from build123d import *

# Parameters (mm, degrees)
F0_W      = 25
F0_H      = 25
F1_DEPTH  = 25
F3_DEPTH  = 25
F9_W      = 25
F9_H      = 25
F10_DEPTH = 25
F11_R     = 5
F12_R     = 5


with BuildPart() as f1:
    # F0 (on Top) → F1 (new body)
    with BuildSketch(Plane.XY):
        Polygon((38.8634320385, -116.9341091547), (38.8634320385, -141.9341091547), (288.8634320385, -141.9341091547), (288.8634320385, 183.0658908453), (38.8634320385, 183.0658908453), (38.8634320385, 158.0658908453), (38.8634320385, 133.0658908453), (38.8634320385, 108.0658908453), (38.8634320385, 83.0658908453), (38.8634320385, 58.0658908453), (38.8634320385, 33.0658908453), (38.8634320385, 8.0658908453), (38.8634320385, -16.9341091547), (38.8634320385, -41.9341091547), (38.8634320385, -66.9341091547), (38.8634320385, -91.9341091547), align=None)
        with Locations((26.3634320385, -129.4341091547)):
            Rectangle(F0_W, F0_H)
        with Locations((26.3634320385, -79.4341091547)):
            Rectangle(F0_W, F0_H)
        with Locations((26.3634320385, -29.4341091547)):
            Rectangle(F0_W, F0_H)
        with Locations((26.3634320385, 20.5658908453)):
            Rectangle(F0_W, F0_H)
        with Locations((26.3634320385, 70.5658908453)):
            Rectangle(F0_W, F0_H)
        with Locations((26.3634320385, 120.5658908453)):
            Rectangle(F0_W, F0_H)
        with Locations((26.3634320385, 170.5658908453)):
            Rectangle(F0_W, F0_H)
    extrude(amount=F1_DEPTH)

    # F2 (on face) → F3 (cut)
    with BuildSketch(Plane.XZ.offset(141.9341091547)):
        Polygon((208.8634320385, 25), (203.8634320385, 0), (228.8634320385, 0), (223.8634320385, 25), align=None)
    extrude(amount=-F3_DEPTH, mode=Mode.SUBTRACT)

    # F8: F1 across plane


with BuildPart() as f1_1:
    add(f1.part)
    add(f1.part.mirror(Plane(origin=(288.8634320385, 20.5658908453, 0), x_dir=(0, 0, 1), z_dir=(0, 1, 0))), mode=Mode.INTERSECT)

    # F9 (on face) → F10 (cut)
    with BuildSketch(Plane(origin=(0, 0, 0), x_dir=(1, 0, 0), z_dir=(0, 0, -1))):
        with Locations((183.8634320385, -145.5658908453)):
            Rectangle(F9_W, F9_H)
        with Locations((183.8634320385, -95.5658908453)):
            Rectangle(F9_W, F9_H)
        with Locations((183.8634320385, -45.5658908453)):
            Rectangle(F9_W, F9_H)
        with Locations((183.8634320385, 4.4341091547)):
            Rectangle(F9_W, F9_H)
        with Locations((183.8634320385, 54.4341091547)):
            Rectangle(F9_W, F9_H)
        with Locations((183.8634320385, 104.4341091547)):
            Rectangle(F9_W, F9_H)
    extrude(amount=-F10_DEPTH, mode=Mode.SUBTRACT)

    # F11
    f11_edges = [f1_1.edges().sort_by_distance(p)[0] for p in [
        (108.863432, -141.934109, 0),
        (111.363432, -141.934109, 25),
        (256.363432, -141.934109, 25),
        (258.863432, -141.934109, 0),
    ]]
    fillet(f11_edges, radius=F11_R)

    # F12
    f12_edges = [f1_1.edges().sort_by_distance(p)[0] for p in [
        (111.363432, 183.065891, 25),
        (108.863432, 183.065891, 0),
        (258.863432, 183.065891, 0),
        (256.363432, 183.065891, 25),
    ]]
    fillet(f12_edges, radius=F12_R)


solid = f1_1.part
Design review of the part built by this model. Coordinates are the model's own, in mm. A direction names the side the tool comes from. Coordinates: 2 decimals unless noted, no trailing zeros. Loops run counter-clockwise (first coordinate to the right, second up) from the corner with the lowest first, then second, coordinate; pieces in that order, holes last. Notation, with made-up numbers: (-6.5, 35.5) -> (27.5, 35.5) arc R31 cw to (27.5, 72.5) -> close; hole circle Ø8 at (-19.75, 78.5). An arc over 180 degrees is marked (long way). Use a Markdown table: item, result. Add a question column.
Item 1: We need section B-B, the plane x = 34. Count the separate pieces of the cut face and the enclosed holes in it, and give its area (3 significant figures).
Item 2: Machinability: for faces 1 (the flat face through (196.363, 96, 12)), 2 (the flat face through (26, 108.066, 12)), 3 (the flat face through (149, 23, 25)), which of the approach directions +Z, -Z, +X, -X, +Y, -Y give a long, thin tool a straight path to every point of the face, cutting with its end or side? Answer none if there is none.
Item 3: Wall thickness on L1, parallel to X at y = -64, z = 15.5; L2, parallel to X at y = 159, z = 20.25; L3, parallel to Y at x = 215.5, z = 4.5: over which ranges is each line inside the solid? List them lowest first. Write a range as from..to.
Item 4: Clearance check with flat-ended pins moving along their axes: P1, Ø1.5, axis at x = 193.5, z = 4.5, coming from the -Y side; P2, Ø12.5, axis at y = -104.5, z = 10, coming from the -X side. State where each tip first meets the part, or that it passes through.
Item 5: We need section A-A, the plane y = -47.5. Write out the cut boundary in (x, z).
Item 6: The part is to be moulded in two halves that separate along X. For faces 4 (the flat face through (184, 133.066, 12)), 5 (the flat face through (256, -141.934, 12)), 6 (the flat face through (38.863, -4, 12)), 7 (the flat face through (184, 58.066, 12)), say which applies: +X half, -X half, draft (parallel to the pull), parting line (faces both ways), or undercut.
Numbers:
| question | item | result |
|---|---|---|
| 1 | separate pieces | 7 |
| 1 | enclosed holes | 0 |
| 1 | area | 4,350 mm^2 |
| 2 | face 1 | +Z, -Z |
| 2 | face 2 | +Z, -Z, -X |
| 2 | face 3 | +Z, +X, -X, +Y, -Y |
| 3 | L1 | x = 38.86..171.36, 196.36..288.86 |
| 3 | L2 | x = 13.86..207.91, 224.81..288.86 |
| 3 | L3 | y = -116.93..158.07 |
| 4 | P1 | stops at y = -141.93 |
| 4 | P2 | stops at x = 38.86 |
| 5 | outline | (38.86, 0) -> (171.36, 0) -> (171.36, 25) -> (38.86, 25) -> close; (196.36, 0) -> (288.86, 0) -> (288.86, 25) -> (196.36, 25) -> close |
| 6 | face 4 | undercut |
| 6 | face 5 | draft |
| 6 | face 6 | -X half |
| 6 | face 7 | undercut |
